Check sheet for the modelled part. Datum: model origin and axes. Units: mm. Face numbers are marked on the shaded views. Round coordinates to 2 decimals unless told otherwise and drop trailing zeros. Order: outer loops, then holes, each group sorted by start corner. A loop starts at its lowest first (then second) coordinate and runs counter-clockwise, first axis right, second up.
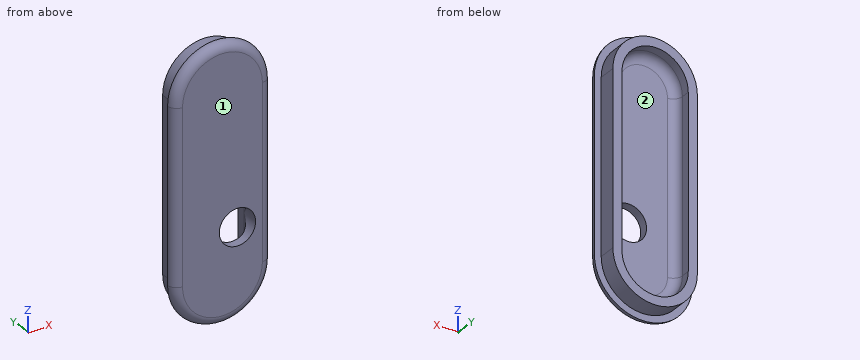
Autodesk Inventor part; units mm, degrees
ref_plane "YZ Plane" through (0, 0, 0) normal (1, 0, 0) x (0, 1, 0)
ref_plane "XZ Plane" through (0, 0, 0) normal (0, 1, 0) x (-1, 0, 0)
ref_plane "XY Plane" through (0, 0, 0) normal (0, 0, 1) x (1, 0, 0)
sketch "Skizze1" plane through (0, 0, 0) normal (0, 1, 0) x (-1, 0, 0)
  line L0 (0, 19) -> (0, -19) construction
  line L1 (-9.3, 19) -> (-9.3, -19)
  line L2 (9.3, -19) -> (9.3, 19)
  arc A0 (9.3, 19) -> (-9.3, 19) centre (0, 19) ccw
  arc A1 (-9.3, -19) -> (9.3, -19) centre (0, -19) ccw
  line L3 (0, 19) -> (0, -19) construction
  line L4 (-10.8, 19) -> (-10.8, -19)
  line L5 (10.8, -19) -> (10.8, 19)
  arc A2 (10.8, 19) -> (-10.8, 19) centre (0, 19) ccw
  arc A3 (-10.8, -19) -> (10.8, -19) centre (0, -19) ccw
  point P0 (0, 0)
  dimension "d0" = 19
  dimension "d1" = 18.6
  dimension "d2" = 1.5
extrude "Extrusion1" add sketch "Skizze1" along normal blind 4 contours A0 L2 A1 L1
extrude "Extrusion2" add sketch "Skizze1" against normal blind 2 contours A0 L2 A1 L1 | A2 L5 A3 L4
fillet "Rundung1" radius 2 4 edges at (-10.8, -2, 0) (0, -2, -29.8) (10.8, -2, 0) (0, -2, 29.8)
sketch "Skizze2" plane through (0, 4, 0) normal (0, 1, 0) x (1, 0, 0)
  line L0 (0, -19) -> (0, 19) construction
  line L1 (-7.3, -19) -> (-7.3, 19)
  line L2 (7.3, 19) -> (7.3, -19)
  arc A0 (-7.3, -19) -> (7.3, -19) centre (0, -19) ccw
  arc A1 (7.3, 19) -> (-7.3, 19) centre (0, 19) ccw
  arc A2 (9.3, 19) -> (-9.3, 19) centre (0, 19) ccw
  line L3 (9.3, -19) -> (9.3, 19)
  point P0 (0, 0)
  dimension "d8" = 2
extrude "Extrusion3" cut sketch "Skizze2" against normal blind 4
fillet "Rundung2" radius 2 4 edges at (0, 0, 26.3) (-7.3, 0, 0) (0, 0, -26.3) (7.3, 0, 0)
sketch "Skizze3" plane through (0, 0, 0) normal (0, 1, 0) x (1, 0, 0)
  circle A0 centre (3.3, 10) radius 4
  line L0 (7.3, 19) -> (7.3, -19)
  point P0 (0, 0)
  dimension "d12" = 8
  dimension "d13" = 10
extrude "Extrusion4" cut sketch "Skizze3" along normal mid plane 4
equation "\"G_L\" = 0"
equation "\"G_H\" = 0"
equation "\"G_B\" = 0"
properties part number "Batterycase_deckel" material "GEDA Stahl"
1) Gauge pin test, flat ends, axial feed: pin 1 (1.5 mm diameter, centred on x = 7, y = -1.5, fed in from +Z); pin 2 (1.6 mm diameter, centred on y = 2.5, z = -4, fed in from +X); pin 3 (8.5 mm diameter, centred on x = 1.5, z = -7.5, fed in from +Y). Record the tip position at first contact, or that the pin passes through.
2) Draft check along Z on the marked faces 1 and 2. Enter one of: pulls with the +Z half, pulls with the -Z half, needs draft (parallel to the pull), parting line crosses it, or undercut.
3) Scan lines: line 1 (X direction, y = 2.25, z = -3); line 2 (X direction, y = -0.3, z = -10); line 3 (Z direction, x = 0.25, y = 2.75). Record each from-to range of solid material in increasing order.
4) Sectioned sample at B-B on y = 1. Record the cut outline in (x, z), and give its area (3 significant figures).
Values found:
1. pin 1: stops at z = 27.33
1. pin 2: stops at x = 9.3
1. pin 3: stops at y = 0.04
2. face 1: needs draft
2. face 2: undercut
3. line 1: x = -9.3 to -7.3, 7.3 to 9.3
3. line 2: x = -10.78 to -0.7, 7.3 to 10.78
3. line 3: z = -28.3 to -26.3, 26.3 to 28.3
4. outline: (-9.3, -19) arc R9.3 ccw to (9.3, -19) - (9.3, 19) arc R9.3 ccw to (-9.3, 19) - close; hole (-7.03, -19) arc R7.03 ccw to (7.03, -19) - (7.03, -11.44) arc R4 ccw to (7.03, -8.56) - (7.03, 19) arc R7.03 ccw to (-7.03, 19) - close
4. area: 288 mm2
